```python
from build123d import *

# Parameters (mm, degrees)
F1_DEPTH = 304.8
F2_R     = 12.7


with BuildPart() as f1:
    # F0 (on Top) → F1 (new body)
    with BuildSketch(Plane.XY):
        Polygon((0, 52.552884), (0, 0), (22.225, 0), (22.225, 38.1), (53.975, 38.1), (53.975, 0), (76.2, 0), (76.2, 482.6), (53.975, 482.6), (53.975, 444.5), (22.225, 444.5), (22.225, 482.6), (0, 482.6), (0, 430.047116), (22.225, 430.047116), (53.975, 430.047116), (53.975, 52.552884), (22.225, 52.552884), align=None)
    extrude(amount=F1_DEPTH)

    # F2
    f2_edges = [f1.edges().sort_by_distance(p)[0] for p in [
        (53.975, 430.047116, 152.4),
        (53.975, 52.552884, 152.4),
    ]]
    fillet(f2_edges, radius=F2_R)


solid = f1.part
```
CAD build for the part. Positions are in the model's coordinates, mm. A direction names the side the tool comes from. Coordinates: 2 decimals unless noted, no trailing zeros. Write each loop counter-clockwise with the first axis right and the second up, starting at its lowest first coordinate (ties: lowest second). Pieces come first, ordered by that corner, then holes.
(1) Cut at D-D, the plane x = 36.5. List the corners of the cut face in (y, z).
(2) Drill centre lines: probe 1 along X at (y, z) = (445, 12) (3 decimals); probe 2 along Y at (x, z) = (34, 98); probe 3 along Y at (x, z) = (7, 98). Where is each one in solid material? Low to high.
(3) 3-axis set-ups, long thin cutter, end or side, ignore diameter. For faces 1 (the face through (54.5, 244.7, 0)), 2 (the face through (11, 0, 150)), 3 (the face through (53.975, 464, 150)), 4 (the face through (22.225, 19, 150)), 5 (the face through (21, 52.553, 150)): which of +Z, -Z, +X, -X, +Y, -Y reach the whole face in a straight line?
(4) Cut at C-C, the plane y = 360.5. List the corners of the cut face in (x, z) (3 decimals).
(5) Cut at B-B, the plane z = 45. List the corners of the cut face in (x, y) (3 decimals).
(6) Two-plate mould, pull along X, no slides. Class faces 6 (the face through (50.156, 426.426, 154.534)), 7 (the face through (38, 38.1, 150)), 8 (the face through (11, 482.6, 150)): +X half, -X half, draft (parallel to the pull), parting line (faces both ways), or undercut.
(7) Flat gauge pins, fed straight in: pin 1 (9.5 mm diameter, centred on x = 44.5, z = 117, fed in from +Y); pin 2 (19 mm diameter, centred on y = 24.5, z = 167, fed in from -X); pin 3 (8 mm diameter, centred on y = 121, z = 101.5, fed in from -X) (3 decimals); pin 4 (8 mm diameter, centred on x = 43.5, z = 238.5, fed in from -Y). Where does each tip first touch, or does it go through?
(8) Cut at A-A, the plane x = 10. List the corners of the cut face in (y, z).
Geometry says:
1. outline: (38.1, 0) - (52.55, 0) - (52.55, 304.8) - (38.1, 304.8) - close; (430.05, 0) - (444.5, 0) - (444.5, 304.8) - (430.05, 304.8) - close
2. probe 1: x = 0 to 22.225, 53.975 to 76.2
2. probe 2: y = 38.1 to 52.55, 430.05 to 444.5
2. probe 3: y = 0 to 52.55, 430.05 to 482.6
3. face 1: -Z, +X, -X, +Y, -Y
3. face 2: +Z, -Z, +X, -X, -Y
3. face 3: +Z, -Z, +Y
3. face 4: +Z, -Z, -Y
3. face 5: +Z, -Z, -X
4. outline: (53.975, 0) - (76.2, 0) - (76.2, 304.8) - (53.975, 304.8) - close
5. outline: (0, 0) - (22.225, 0) - (22.225, 38.1) - (53.975, 38.1) - (53.975, 0) - (76.2, 0) - (76.2, 482.6) - (53.975, 482.6) - (53.975, 444.5) - (22.225, 444.5) - (22.225, 482.6) - (0, 482.6) - (0, 430.047) - (41.275, 430.047) arc R12.7 cw to (53.975, 417.347) - (53.975, 65.253) arc R12.7 cw to (41.275, 52.553) - (0, 52.553) - close
6. face 6: -X half
6. face 7: undercut
6. face 8: draft
7. pin 1: stops at y = 444.5
7. pin 2: stops at x = 0
7. pin 3: stops at x = 53.975
7. pin 4: stops at y = 38.1
8. outline: (0, 0) - (52.55, 0) - (52.55, 304.8) - (0, 304.8) - close; (430.05, 0) - (482.6, 0) - (482.6, 304.8) - (430.05, 304.8) - close
